from build123d import *

# Parameters (mm, degrees)
SKETCH_1_W      = 200
SKETCH_1_H      = 150
EXTRUDE_1_DEPTH = 100
SKETCH_2_R      = 10
EXTRUDE_2_DEPTH = 5


with BuildPart() as part:
    # 草图1 → 凸台-拉伸1 (new, symmetric)
    with BuildSketch(Plane.XY):
        Rectangle(SKETCH_1_W, SKETCH_1_H)
    extrude(amount=EXTRUDE_1_DEPTH, both=True)

    # 草图2 → 凸台-拉伸2 (add)
    with BuildSketch(Plane.XY.offset(100)):
        with Locations(Location((0, 9.852813742, 0), (0, 0, 180))):
            Circle(SKETCH_2_R)
        with Locations(Location((84.852813742, -50.756338931, 0), (0, 0, 180))):
            Circle(SKETCH_2_R)
    extrude_2 = extrude(amount=EXTRUDE_2_DEPTH)

    # 镜向1: 凸台-拉伸2 across plane
    add(extrude_2.mirror(Plane.XY))


solid = part.part
Verification items for the finished model (mm, model axes). A direction names the side the tool comes from. Coordinates: 2 decimals unless noted, no trailing zeros. Write each loop counter-clockwise with the first axis right and the second up, starting at its lowest first coordinate (ties: lowest second). Pieces come first, ordered by that corner, then holes. Notation, with made-up numbers: (-34.5, -12.75) -> (-22.5, -12.75) arc R19 ccw to (-22.5, 0.25) -> close; hole circle Ø10 at (15, 0). An arc over 180 degrees is marked (long way). One line per item, written item: value. Start each with the question number.
Q1. Thickness scan on L1, parallel to Z at x = -58.5, y = -16. Record the ranges inside material, lowest first. Write a range as from..to.
Q2. Cross-section at C-C on x = -52.5. Enter the section's corners in (y, z), and give its area (3 significant figures).
Q3. Cross-section at A-A on x = 0. Enter the section's corners in (y, z).
Q4. Go/stop test with a flat-tipped pin: P1, Ø1.5, axis at x = 26, y = -54, coming from the +Z side. Record where the tip stops, or that it passes through.
Q5. Cross-section at B-B on y = -6. Enter the section's corners in (x, z).
Q6. Access from +Z, -Z, +X, -X, +Y, -Y to the whole of each face (thin tool, end or side, straight path). Record for faces 1 (the cylindrical face through (75.615, -46.926, -102.465)), 2 (the cylindrical face through (2.168, 19.615, 102.465)), 3 (the flat face through (-1, 75, 1)).
Checked values:
1. L1: z = -100..100
2. outline: (-75, -100) -> (75, -100) -> (75, 100) -> (-75, 100) -> close
2. area: 30,000 mm²
3. outline: (-75, -100) -> (-0.15, -100) -> (-0.15, -105) -> (19.85, -105) -> (19.85, -100) -> (75, -100) -> (75, 100) -> (19.85, 100) -> (19.85, 105) -> (-0.15, 105) -> (-0.15, 100) -> (-75, 100) -> close
4. P1: stops at z = 100
5. outline: (-100, -100) -> (100, -100) -> (100, 100) -> (-100, 100) -> close
6. face 1: -Z
6. face 2: +Z
6. face 3: +Z, -Z, +X, -X, +Y
